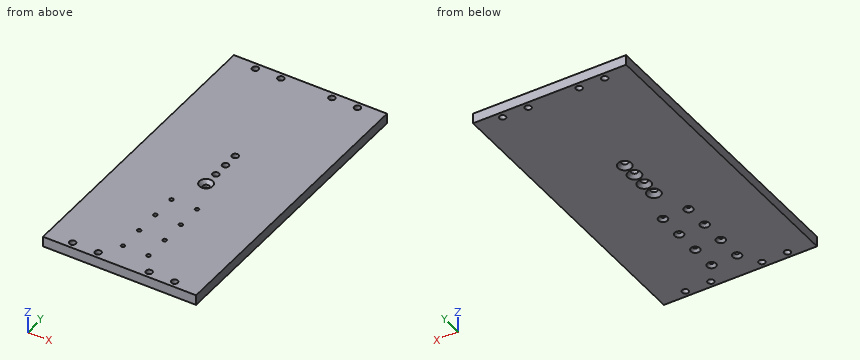
Autodesk Inventor part; units mm, degrees
ref_plane "YZ Plane" through (0, 0, 0) normal (1, 0, 0) x (0, 1, 0)
ref_plane "XZ Plane" through (0, 0, 0) normal (0, 1, 0) x (-1, 0, 0)
ref_plane "XY Plane" through (0, 0, 0) normal (0, 0, 1) x (1, 0, 0)
sketch "Szkic1" plane through (0, 0, 0) normal (0, 0, 1) x (1, 0, 0)
  line L0 (-50, -65) -> (50, -65)
  line L1 (50, -65) -> (50, 65)
  line L2 (50, 65) -> (-50, 65)
  line L3 (-50, 65) -> (-50, -65)
  line L4 (-50, -65) -> (50, 65) construction
  line L5 (50, -65) -> (-50, 65) construction
  point P0 (0, 0)
  dimension "d0" = 100
  dimension "d1" = 130
extrude "Wyciągnięcie proste1" add sketch "Szkic1" along normal blind 8
sketch "Szkic7" plane through (-50, 65, 0) normal (0, 1, 0) x (1, 0, 0)
  line L0 (100, 0) -> (0, 0)
  line L1 (0, 0) -> (0, -8)
  line L2 (100, -8) -> (0, -8)
  line L3 (100, 0) -> (100, -8)
  point P0 (50, 0)
extrude "Wyciągnięcie proste6" add sketch "Szkic7" along normal blind 45
sketch "Szkic9" plane through (0, 0, 0) normal (0, 0, -1) x (-1, 0, 0)
  circle A0 centre (-10, -5) radius 1.5
  circle A1 centre (-10, 15) radius 1.5
  circle A2 centre (10, -5) radius 1.5
  circle A3 centre (10, 15) radius 1.5
  circle A4 centre (-10, -45) radius 1.5
  circle A5 centre (-10, -25) radius 1.5
  circle A6 centre (10, -45) radius 1.5
  circle A7 centre (10, -25) radius 1.5
  line L0 (50, -65) -> (-50, -65)
  line L1 (50, -65) -> (50, 110)
  line L2 (-50, 110) -> (50, 110)
  line L3 (-50, -65) -> (-50, 110)
  circle A8 centre (-10, -45) radius 1.5
  circle A9 centre (-10, -55) radius 1.5
  line L4 (-10, -55) -> (-10, -45)
  point P0 (0, 10)
  dimension "d119" = 10
hole "Otwór2" at (10, 15, 0) at (-10, 15, 0) at (-10, -5, 0) at (10, -5, 0) at (10, -25, 0) at (-10, -25, 0) at (-10, -45, 0) at (10, -45, 0) direction (0, 0, 1) diameter 3 end through all countersink diameter 7 countersink angle 90
sketch "Szkic10" plane through (50, -65, 8) normal (1, 0, 0) x (0, 0, -1)
  line L0 (8, 0) -> (8, 175)
  line L1 (0, 175) -> (8, 175)
  line L2 (0, 0) -> (0, 175)
  line L3 (8, 0) -> (0, 0)
  point P0 (8, 65)
sketch "Szkic11" plane through (-50, -65, 0) normal (-1, 0, 0) x (0, 0, 1)
  line L0 (0, 0) -> (0, 175)
  line L1 (0, 0) -> (8, 0)
  line L2 (8, 0) -> (8, 175)
  line L3 (0, 175) -> (8, 175)
  point P0 (0, 65)
extrude "Wyciągnięcie proste8" add sketch "Szkic11" along normal blind 10
extrude "Wyciągnięcie proste9" add sketch "Szkic10" along normal blind 10
sketch "Szkic14" plane through (0, 0, 8) normal (0, 0, 1) x (1, 0, 0)
  line L0 (60, -75) -> (-60, -75)
  line L1 (-60, -65) -> (-60, 110)
  line L2 (60, 110) -> (60, -65)
  line L3 (-60, -65) -> (-60, -55)
  line L4 (-60, 110) -> (-60, -65)
  line L5 (-60, -55) -> (60, -55)
  line L6 (-60, -55) -> (-60, -60)
  line L7 (-60, -60) -> (60, -60)
  line L8 (-60, -65) -> (-40, -65)
  line L9 (-60, -75) -> (60, -75)
  line L10 (-40, -65) -> (-40, -55)
  line L11 (-40, -65) -> (-20, -65)
  line L12 (-20, -65) -> (-20, -55)
  line L13 (-20, -65) -> (20, -65)
  line L14 (20, -65) -> (20, -55)
  line L15 (20, -65) -> (40, -65)
  line L16 (40, -65) -> (40, -55)
  circle A0 centre (-40, -60) radius 2.5
  circle A1 centre (-20, -60) radius 2.5
  circle A2 centre (20, -60) radius 2.5
  circle A3 centre (40, -60) radius 2.5
  line L17 (-60, -65) -> (-60, -55)
  point P0 (0, 0)
  dimension "d84" = 20
  dimension "d85" = 5
  dimension "d87" = 20
  dimension "d89" = 20
  dimension "d90" = 5
  dimension "d91" = 5
  dimension "d92" = 5
  dimension "d93" = 5
  dimension "d105" = 20
  dimension "d120" = 10
  dimension "d121" = 20
hole "Otwór5" at (-40, -60, 8) at (-20, -60, 8) at (20, -60, 8) at (40, -60, 8) direction (0, 0, -1) diameter 5 end through all
sketch "Szkic16" plane through (-50, 110, 0) normal (0, 1, 0) x (1, 0, 0)
  line L0 (-10, 0) -> (110, 0)
  line L1 (-10, -8) -> (-10, 0)
  line L2 (110, -8) -> (-10, -8)
  line L3 (110, 0) -> (110, -8)
  point P0 (50, 0)
extrude "Wyciągnięcie proste12" add sketch "Szkic16" along normal blind 61
sketch "Szkic17" plane through (0, 0, 0) normal (0, 0, -1) x (-1, 0, 0)
  line L0 (60, 161) -> (-60, 161)
  line L1 (-60, 346) -> (-60, 161)
  line L2 (60, 346) -> (60, 161)
  line L3 (-60, 161) -> (-60, 171)
  line L4 (-60, 346) -> (-60, 161)
  line L5 (-60, 171) -> (60, 171)
  line L6 (-60, 171) -> (-60, 166)
  line L7 (-60, 166) -> (60, 166)
  line L8 (-60, 161) -> (-40, 161)
  line L9 (-60, 161) -> (60, 161)
  line L10 (-40, 161) -> (-40, 171)
  line L11 (-40, 161) -> (-20, 161)
  line L12 (-20, 161) -> (-20, 171)
  line L13 (-20, 161) -> (20, 161)
  line L14 (20, 161) -> (20, 171)
  line L15 (20, 161) -> (40, 161)
  line L16 (40, 161) -> (40, 171)
  circle A0 centre (-40, 166) radius 2.5
  circle A1 centre (-20, 166) radius 2.5
  circle A2 centre (20, 166) radius 2.5
  circle A3 centre (40, 166) radius 2.5
  line L17 (-60, 171) -> (60, 171)
  point P0 (0, 0)
  point P1 (0, 236)
  dimension "d106" = 10
  dimension "d107" = 5
  dimension "d108" = 20
  dimension "d109" = 20
  dimension "d110" = 20
  dimension "d111" = 5
  dimension "d112" = 5
  dimension "d113" = 5
  dimension "d114" = 5
  dimension "d115" = 20
extrude "Wyciągnięcie proste13" cut sketch "Szkic17" against normal up to next contours A3 L7 L16 | L16 L7 A3 | L7 L16 A3 | A2 L7 L14 | L14 L7 A2 | L7 A3 L16 | A1 L7 L12 | L12 L7 A1 | L14 A2 L7 | L7 A2 L14 | A0 L7 L10 | L10 L7 A0 | L12 A1 L7 | L7 A1 L12 | L10 A0 L7 | L7 A0 L10
sketch "Szkic18" plane through (0, 0, 8) normal (0, 0, 1) x (1, 0, 0)
  line L0 (10, 30) -> (10, 90)
  line L1 (10, 90) -> (-10, 90)
  line L2 (-10, 90) -> (-10, 30)
  line L3 (10, 30) -> (-10, 30)
  line L4 (-10, 30) -> (-10, 90)
  line L5 (-10, 30) -> (0, 30)
  line L6 (0, 30) -> (0, 90)
  line L7 (10, 90) -> (-10, 90)
  line L8 (0, 30) -> (0, 42)
  line L9 (0, 42) -> (0, 54)
  line L10 (0, 54) -> (0, 66)
  line L11 (0, 66) -> (0, 78)
  circle A0 centre (0, 42) radius 2.5
  circle A1 centre (0, 54) radius 2.5
  circle A2 centre (0, 66) radius 2.5
  circle A3 centre (0, 78) radius 2.5
  line L12 (-60, 171) -> (60, 171)
  line L13 (60, -65) -> (60, 171)
  line L14 (60, -65) -> (60, 171)
  line L15 (60, 171) -> (60, 90)
  line L16 (60, 90) -> (0, 90)
  line L17 (-60, -65) -> (-60, 171)
  line L18 (0, 171) -> (0, -65)
  line L19 (60, -65) -> (-60, -65)
  point P0 (0, 0)
  point P1 (13, 60)
  dimension "d122" = 10
  dimension "d123" = 12
  dimension "d124" = 12
  dimension "d125" = 12
  dimension "d126" = 12
  dimension "d127" = 5
  dimension "d128" = 5
  dimension "d129" = 5
  dimension "d130" = 5
  dimension "d131" = 81
extrude "Wyciągnięcie proste14" cut sketch "Szkic18" against normal up to next contours A0 L6 | L6 A0 | A3 L6 | L6 A3 | A1 L6 | L6 A1 | A2 L6 | L6 A2
hole "Otwór6" at (0, 78, 0) direction (0, 0, 1) diameter 5 end through all countersink diameter 10.5 countersink angle 90
hole "Otwór7" at (0, 66, 0) direction (0, 0, 1) diameter 5 end through all countersink diameter 10.5 countersink angle 90
hole "Otwór8" at (0, 42, 8) direction (0, 0, -1) diameter 5 end through all countersink diameter 10.5 countersink angle 90
hole "Otwór9" at (0, 54, 0) direction (0, 0, 1) diameter 5 end through all countersink diameter 10.5 countersink angle 90
hole "Otwór10" at (0, 42, 0) direction (0, 0, 1) diameter 5 end through all countersink diameter 10.5 countersink angle 90
properties part number "Wspornik pionowy osi Z"
Work out the finished part from the listing and answer in its coordinate system (mm). Coordinates: 2 decimals unless noted, no trailing zeros. Write each loop counter-clockwise with the first axis right and the second up, starting at its lowest first coordinate (ties: lowest second). Pieces come first, ordered by that corner, then holes. Notation, with made-up numbers: (11.25, 68) - (56.25, 68) arc R14 ccw to (56.25, 92) - close; hole circle Ø3 at (28.25, 47.25). An arc over 180 degrees is marked (long way). One line per question, with ' | ' between items.
1) Find section A-A, the plane x = 20. Determine the outline of the cut face in (y, z).
Checks:
outline: (-65, 0) - (-62.5, 0) - (-62.5, 8) - (-65, 8) - close; (-57.5, 0) - (163.5, 0) - (163.5, 8) - (-57.5, 8) - close; (168.5, 0) - (171, 0) - (171, 8) - (168.5, 8) - close
2) Find section C-C, the plane y = 166. Determine the outline of the cut face in (x, z), and give its area (3 significant figures).
Checks:
outline: (-60, 0) - (-42.5, 0) - (-42.5, 8) - (-60, 8) - close; (-37.5, 0) - (-22.5, 0) - (-22.5, 8) - (-37.5, 8) - close; (-17.5, 0) - (17.5, 0) - (17.5, 8) - (-17.5, 8) - close; (22.5, 0) - (37.5, 0) - (37.5, 8) - (22.5, 8) - close; (42.5, 0) - (60, 0) - (60, 8) - (42.5, 8) - close | area: 800 mm2
3) Find section D-D, the plane y = 42. Determine the outline of the cut face in (x, z).
Checks:
outline: (-60, 0) - (-5.25, 0) - (-2.5, 2.75) - (-2.5, 5.25) - (-5.25, 8) - (-60, 8) - close; (2.5, 2.75) - (5.25, 0) - (60, 0) - (60, 8) - (5.25, 8) - (2.5, 5.25) - close
4) Consider probe 1 along Y at (x, z) = (20, 4.25); probe 2 along X at (y, z) = (15, 3.35); probe 3 along X at (y, z) = (-60, 4.75). Determine where each line is inside the solid, lowest interval first. Write a range as [from, to].
Checks:
probe 1: [-65, -62.5], [-57.5, 163.5], [168.5, 171] | probe 2: [-60, -11.5], [-8.5, 8.5], [11.5, 60] | probe 3: [-60, -42.5], [-37.5, -22.5], [-17.5, 17.5], [22.5, 37.5], [42.5, 60]
5) Find section B-B, the plane y = 78. Determine the outline of the cut face in (x, z), and give its area (3 significant figures).
Checks:
outline: (-60, 0) - (-5.25, 0) - (-2.5, 2.75) - (-2.5, 8) - (-60, 8) - close; (2.5, 2.75) - (5.25, 0) - (60, 0) - (60, 8) - (2.5, 8) - close | area: 912 mm2
6) Flat-ended cylindrical pins translate along their axes: P1, Ø4, axis at x = -10, y = -25, coming from the -Z side; P2, Ø3.5, axis at x = 10, y = -5, coming from the -Z side; P3, Ø6.5, axis at x = 0, y = 42, coming from the -Z side. Find the tip coordinate at first contact, or state that the pin passes through.
Checks:
P1: z = 1.5 | P2: z = 1.75 | P3: z = 2
